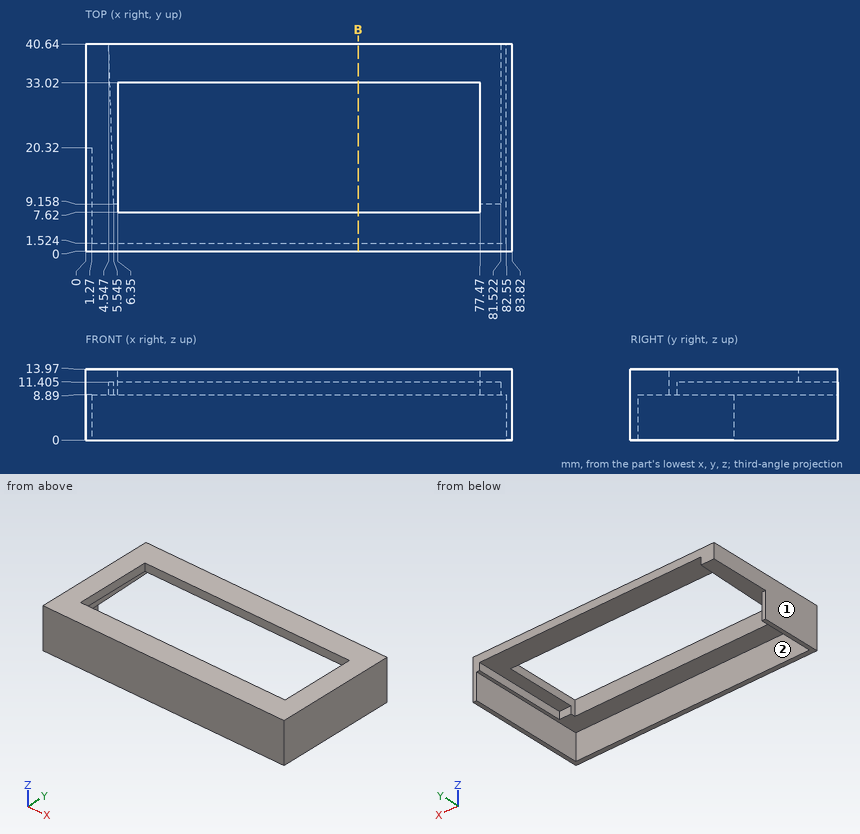
The figure shows three views and two pictorial views of one solid part (mm, origin at its lowest corner). Answer the questions. A direction names the side the tool comes from. Round coordinates to 2 decimals unless told otherwise and drop trailing zeros. Write each loop counter-clockwise with the first axis right and the second up, starting at its lowest first coordinate (ties: lowest second). Pieces come first, ordered by that corner, then holes. Notation, with made-up numbers: M -34,25.25 L 12,25.25 A22 cw 12,63.25 Z; hole C -5,37 d6. An arc over 180 degrees is marked long. Write each question's results on one line, items separated by ' | '. Start each with the question number.
(1) For the marked faces 1 and 2, determine the directions among +Z, -Z, +X, -X, +Y, -Y from which every point of the face is accessible in a straight line to the end or side of a thin tool.
(2) Each of these flat-tipped pins is pushed along its axis until it touches: P1, Ø1.3, axis at x = 80.5, z = 10, coming from the +Y side; P2, Ø8, axis at x = 39.5, z = 3, coming from the +Y side; P3, Ø2.5, axis at y = 30.5, z = 4, coming from the -X side. Where does it stop, or does it pass through?
(3) Find the intervals of material crossed by line 1 (X direction, y = 19.5, z = 5); line 2 (Y direction, x = 8.5, z = 13); line 3 (Y direction, x = 19, z = 5), in increasing order.
(4) The part is cut by section B-B, the plane x = 53.5. Write down the section's boundary in (y, z) (1 decimal).
Worked answers:
1) face 1: +Z, -Z, -X, +Y, -Y | face 2: -Z, +Y
2) P1: stops at y = 9.16 | P2: stops at y = 1.52 | P3: stops at x = 82.55
3) line 1: x = 0 to 1.27, 82.55 to 83.82 | line 2: y = 0 to 7.62, 33.02 to 40.64 | line 3: y = 0 to 1.52
4) outline: M 0,0 L 1.5,0 L 1.5,8.9 L 7.6,8.9 L 7.6,14 L 0,14 Z; M 33,11.4 L 40.6,11.4 L 40.6,14 L 33,14 Z
